from build123d import *

# Parameters (mm, degrees)
F1_DEPTH = 85
F2_R     = 4
F3_DEPTH = 25


with BuildPart() as f1:
    # F0 (on Front) → F1 (new body)
    with BuildSketch(Plane.XZ):
        Polygon((67.613126, -11.305504), (-79.386874, -11.305504), (-93.386874, -11.305504), (-93.386874, -13.305504), (-79.386874, -13.305504), (-79.386874, -49.860391), (67.613126, -49.860391), (67.613126, -13.305504), (81.613126, -13.305504), (81.613126, -11.305504), align=None)
    extrude(amount=F1_DEPTH)

    # F2 (on face) → F3 (cut)
    with BuildSketch(Plane.XY.offset(-11.305504)):
        with Locations((-85.386874, -42.530299)):
            Circle(F2_R)
        with Locations((73.613126, -43.162795)):
            Circle(F2_R)
    extrude(amount=-F3_DEPTH, mode=Mode.SUBTRACT)


solid = f1.part
Model file for the job. Use its own axes, mm. A direction names the side the tool comes from. Give positions to 0.01 mm unless a question says otherwise; leave off trailing zeros. Order: outer loops, then holes, each group sorted by start corner. A loop starts at its lowest first (then second) coordinate and runs counter-clockwise, first axis right, second up. Notation, with made-up numbers: M 27,-6 L 66,-6 A28 cw 66,33 Z; hole C -5,66 d2. An arc over 180 degrees is marked long. Put each result on its own line as item: value. Start each with the question number.
(1) Band-saw the part on A-A on y = -53. Give the cut face in (x, z).
(2) Pin check, flat tips, straight feed: pin 1 Ø8 at (y, z) = (-12.5, -45) entering from +X; pin 2 Ø15.5 at (x, y) = (77.5, -44) entering from -Z. Stop position of each tip, or through.
(3) Band-saw the part on B-B on z = -27. Give the cut face in (x, y), then the cut area to 3 significant figures.
(4) Tool access for faces 4 (the face through (-79.387, -42, -31)), 5 (the face through (-7, 0, -30)), 6 (the face through (78, -42, -13.306)): list every direction of +Z, -Z, +X, -X, +Y, -Y with a clear straight run to the whole face (end or side of a thin tool).
(5) Drill centre line: L1, parallel to X at y = -23, z = -21.5. Where is it in solid material? Low to high. Write a range as [from, to].
(6) Pull direction Y, two halves, no side cores. Call faces 1 (the face through (-7, -42, -49.86)), 2 (the face through (-7, -85, -30)), 3 (the face through (-89.383, -42.354, -12.292)): released by +Y, released by -Y, zero draft, split by the parting line, or undercut.
Results below:
1. outline: M -93.39,-13.31 L -79.39,-13.31 L -79.39,-49.86 L 67.61,-49.86 L 67.61,-13.31 L 81.61,-13.31 L 81.61,-11.31 L -93.39,-11.31 Z
2. pin 1: stops at x = 67.61
2. pin 2: stops at z = -13.31
3. outline: M -79.39,-85 L 67.61,-85 L 67.61,0 L -79.39,0 Z
3. area: 12,500 mm2
4. face 4: -Z, -X, +Y, -Y
4. face 5: +Z, -Z, +X, -X, +Y
4. face 6: -Z, +X, +Y, -Y
5. L1: x = [-79.39, 67.61]
6. face 1: zero draft
6. face 2: released by -Y
6. face 3: undercut
